```python
from build123d import *

# Parameters (mm, degrees)
BOSS_EXTRU_1_DEPTH = 2.5


with BuildPart() as part:
    # Esquisse1 → Boss.-Extru.1 (new body)
    with BuildSketch(Plane(origin=(0, 0, 0), x_dir=(1, 0, 0), z_dir=(0, 1, 0))):
        with BuildLine():
            Line((33.7, 0), (-30.6, 0))
            ThreePointArc((-30.6, 0), (-31.458125453, -2.141027444), (-33.557418398, -3.09671931))
            ThreePointArc((-33.557418398, -3.09671931), (-16.85, -29.185056108), (14.096871608, -30.609936473))
            ThreePointArc((14.096871608, -30.609936473), (15.3, -26.500377356), (19.46054679, -27.513217163))
            ThreePointArc((19.46054679, -27.513217163), (29.929169942, -15.489828488), (33.7, 0))
        make_face()
        with BuildLine():
            ThreePointArc((-33.557418398, 3.09671931), (-31.458125453, 2.141027444), (-30.6, 0))
            Line((-30.6, 0), (33.7, 0))
            ThreePointArc((33.7, 0), (29.929169942, 15.489828488), (19.46054679, 27.513217163))
            ThreePointArc((19.46054679, 27.513217163), (15.3, 26.500377356), (14.096871608, 30.609936473))
            ThreePointArc((14.096871608, 30.609936473), (-16.85, 29.185056108), (-33.557418398, 3.09671931))
        make_face()
    extrude(amount=BOSS_EXTRU_1_DEPTH)


solid = part.part
```
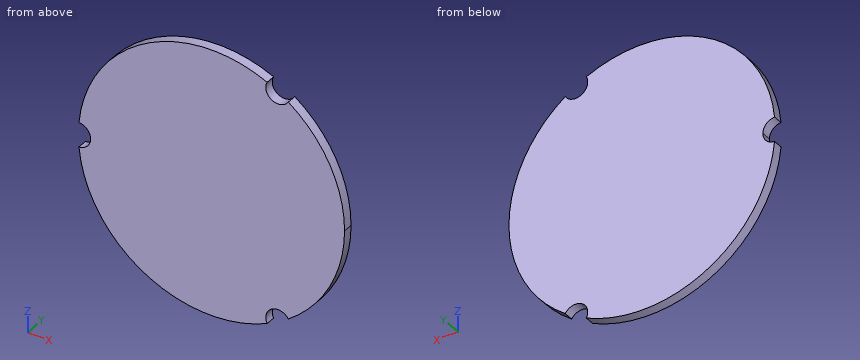
Work out the finished part from the listing and answer in its coordinate system (mm). Round coordinates to 2 decimals unless told otherwise and drop trailing zeros. Loops run counter-clockwise (first coordinate to the right, second up) from the corner with the lowest first, then second, coordinate; pieces in that order, holes last. Notation, with made-up numbers: (-36.5, 68.5) -> (18.5, 68.5) arc R14 ccw to (18.5, 76.5) -> close; hole circle Ø9 at (-28, 85). An arc over 180 degrees is marked (long way). Write each question's results on one line, items separated by ' | '. Start each with the question number.
1. Section A-A (y = 1.3) is taken. Determine the outline of the cut face in (x, z).
2. Section C-C (z = -23.5) is taken. Determine the outline of the cut face in (x, y), plus the area to 3 significant figures.
3. Find the intervals of material crossed by probe 1 along Z at (x, y) = (1, 0.75); probe 2 along X at (y, z) = (0.25, -27); probe 3 along Z at (x, y) = (13.5, 1), in increasing order. Write a range as from..to.
4. Section B-B (x = 16.85) is taken. Determine the outline of the cut face in (y, z), plus the area to 3 significant figures.
5. Given pin 1 Ø6 at (x, z) = (5.5, -5) entering from -Y; pin 2 Ø1.5 at (x, y) = (3, 1) entering from +Z; pin 3 Ø1 at (x, y) = (-7, 1.5) entering from -Z, each flat-ended and moving along its own axis, determine where each tip first touches the part or whether it passes through.
Evaluation:
1) outline: (-33.56, -3.1) arc R33.7 ccw to (14.1, -30.61) arc R3.1 cw to (19.46, -27.51) arc R33.7 ccw to (19.46, 27.51) arc R3.1 cw to (14.1, 30.61) arc R33.7 ccw to (-33.56, 3.1) arc R3.1 cw to start
2) outline: (-24.15, 0) -> (24.15, 0) -> (24.15, 2.5) -> (-24.15, 2.5) -> close | area: 121 mm2
3) probe 1: z = -33.69..33.69 | probe 2: x = -20.17..14.65, 19.05..20.17 | probe 3: z = -30.88..30.88
4) outline: (0, -26.09) -> (2.5, -26.09) -> (2.5, 26.09) -> (0, 26.09) -> close | area: 130 mm2
5) pin 1: stops at y = 0 | pin 2: stops at z = 33.62 | pin 3: stops at z = -33.07
